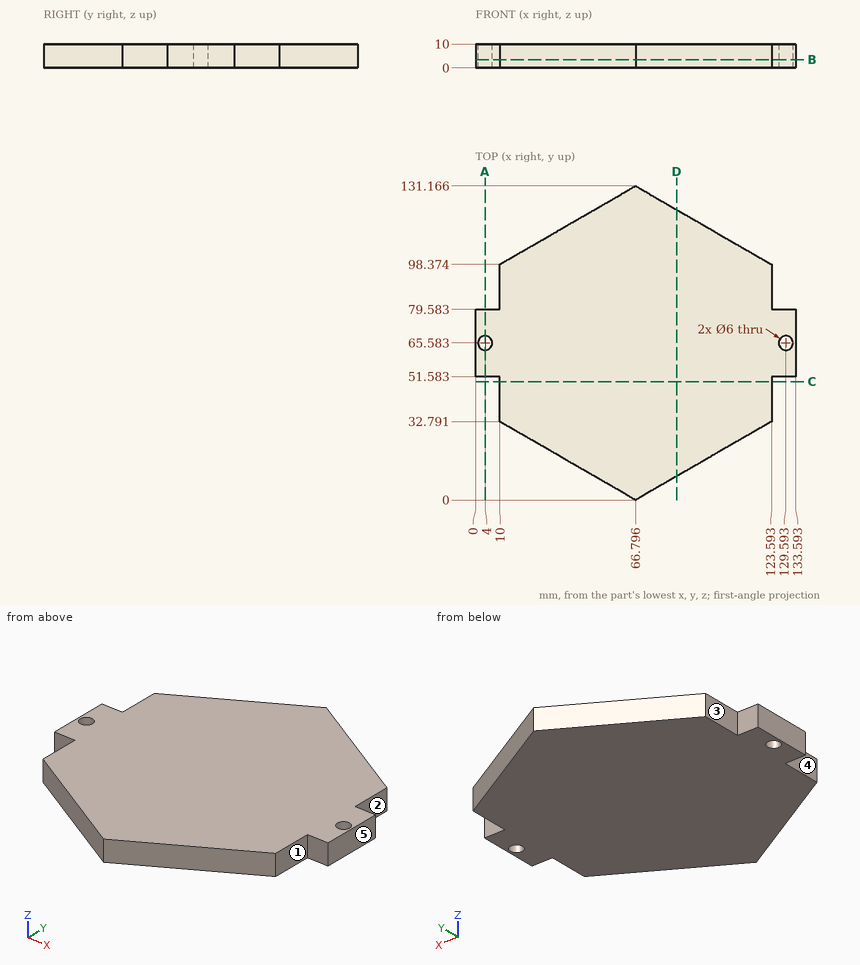
Drawing for the job (mm, zero at the part's lowest x, y, z). A direction names the side the tool comes from. Coordinates: 2 decimals unless noted, no trailing zeros. Loops run counter-clockwise (first coordinate to the right, second up) from the corner with the lowest first, then second, coordinate; pieces in that order, holes last. Notation, with made-up numbers: (-5.5, 45) - (0.5, 45) arc R22 cw to (0.5, 62) - close; hole circle Ø10 at (26.25, 43). An arc over 180 degrees is marked (long way). Use CSV: the item, a comma, the result in double quotes. Start each with the question number.
Q1. Cut at B-B, the plane z = 3.5. List the corners of the cut face in (x, y) (1 decimal), then the cut area to 3 significant figures.
Q2. Cut at D-D, the plane x = 84. List the corners of the cut face in (y, z), then the cut area to 3 significant figures.
Q3. Cut at A-A, the plane x = 4. List the corners of the cut face in (y, z).
Q4. Cut at C-C, the plane y = 49.5. List the corners of the cut face in (x, z).
Q5. Probe probe 1 along X at (y, z) = (65.5, 9.75) (1 decimal); probe 2 along Y at (x, z) = (4, 4.5); probe 3 along X at (y, z) = (67.5, 9.25) (1 decimal). List the from-to ranges inside material, lowest first. Write a range as from..to.
Q6. Drop flat-ended pins along their axis: P1, Ø5, axis at x = 79, z = 5, coming from the +Y side; P2, Ø5, axis at x = 129.59, y = 65.58, coming from the -Z side; P3, Ø3, axis at x = 5, z = 4, coming from the -Y side; P4, Ø5, axis at y = 87.5, z = 5.5, coming from the +X side. Give the stop position or say it passes through.
Q7. 3-axis set-ups, long thin cutter, end or side, ignore diameter. For the marked faces 1, 2, 3, 4 and 5: which of +Z, -Z, +X, -X, +Y, -Y reach the whole face in a straight line?
Here are the results:
1,outline,"(0, 51.6) - (10, 51.6) - (10, 32.8) - (66.8, 0) - (123.6, 32.8) - (123.6, 51.6) - (133.6, 51.6) - (133.6, 79.6) - (123.6, 79.6) - (123.6, 98.4) - (66.8, 131.2) - (10, 98.4) - (10, 79.6) - (0, 79.6) - close; hole circle Ø6 at (4, 65.6); hole circle Ø6 at (129.6, 65.6)"
1,area,"11,700 mm2"
2,outline,"(9.93, 0) - (121.23, 0) - (121.23, 10) - (9.93, 10) - close"
2,area,"1,110 mm2"
3,outline,"(51.58, 0) - (62.58, 0) - (62.58, 10) - (51.58, 10) - close; (68.58, 0) - (79.58, 0) - (79.58, 10) - (68.58, 10) - close"
4,outline,"(10, 0) - (123.59, 0) - (123.59, 10) - (10, 10) - close"
5,probe 1,"0..1, 7..126.6, 132.6..133.6"
5,probe 2,"51.58..62.58, 68.58..79.58"
5,probe 3,"0..1.7, 6.3..127.3, 131.9..133.6"
6,P1,"y = 125.56"
6,P2,"through"
6,P3,"y = 51.58"
6,P4,"x = 123.59"
7,face 1,"+Z, -Z, +X, -Y"
7,face 2,"+Z, -Z, +X, +Y"
7,face 3,"+Z, -Z, -X, +Y"
7,face 4,"+Z, -Z, -X, -Y"
7,face 5,"+Z, -Z, +X, +Y, -Y"
